from build123d import *

# Parameters (mm, degrees)
F0_R     = 63.5
F1_DEPTH = 63.5
F2_R     = 2.776459
F2_R_2   = 2.032
F2_R_3   = 3.5052
F3_DEPTH = 101.6


with BuildPart() as f1:
    # F0 (on Top) → F1 (new body, symmetric)
    with BuildSketch(Plane.XY):
        Circle(F0_R)
    extrude(amount=F1_DEPTH, both=True)

    # F2 (on face) → F3 (cut)
    with BuildSketch(Plane.XY.offset(63.5)):
        with BuildLine():
            ThreePointArc((-3.5052, 0), (0, -3.5052), (3.5052, 0))
            ThreePointArc((3.5052, 0), (0, 3.5052), (-3.5052, 0))
        make_face()
        with Locations((-47.625, 0)):
            Circle(F2_R)
        with BuildLine():
            ThreePointArc((-33.782, 0), (-31.75, -2.032), (-29.718, 0))
            Line((-29.718, 0), (-31.75, 0))
            Line((-31.75, 0), (-33.782, 0))
        make_face()
        with BuildLine():
            Line((-31.75, 0), (-29.718, 0))
            ThreePointArc((-29.718, 0), (-31.75, 2.032), (-33.782, 0))
            Line((-33.782, 0), (-31.75, 0))
        make_face()
        with BuildLine():
            ThreePointArc((-19.3802, 0), (-15.875, -3.5052), (-12.3698, 0))
            Line((-12.3698, 0), (-15.875, 0))
            Line((-15.875, 0), (-19.3802, 0))
        make_face()
        with BuildLine():
            Line((-15.875, 0), (-12.3698, 0))
            ThreePointArc((-12.3698, 0), (-15.875, 3.5052), (-19.3802, 0))
            Line((-19.3802, 0), (-15.875, 0))
        make_face()
        with Locations((-46.002217, -12.326257)):
            Circle(F2_R)
        with Locations((-41.24446, -23.8125)):
            Circle(F2_R)
        with Locations((-33.67596, -33.67596)):
            Circle(F2_R)
        with Locations((-23.8125, -41.24446)):
            Circle(F2_R)
        with Locations((-12.326257, -46.002217)):
            Circle(F2_R)
        with Locations((0, -47.625)):
            Circle(F2_R)
        with Locations((12.326257, -46.002217)):
            Circle(F2_R)
        with Locations((23.8125, -41.24446)):
            Circle(F2_R)
        with Locations((33.67596, -33.67596)):
            Circle(F2_R)
        with Locations((41.24446, -23.8125)):
            Circle(F2_R)
        with Locations((46.002217, -12.326257)):
            Circle(F2_R)
        with Locations((47.625, 0)):
            Circle(F2_R)
        with Locations((46.002217, 12.326257)):
            Circle(F2_R)
        with Locations((41.24446, 23.8125)):
            Circle(F2_R)
        with Locations((33.67596, 33.67596)):
            Circle(F2_R)
        with Locations((23.8125, 41.24446)):
            Circle(F2_R)
        with Locations((12.326257, 46.002217)):
            Circle(F2_R)
        with Locations((0, 47.625)):
            Circle(F2_R)
        with Locations((-12.326257, 46.002217)):
            Circle(F2_R)
        with Locations((-23.8125, 41.24446)):
            Circle(F2_R)
        with Locations((-33.67596, 33.67596)):
            Circle(F2_R)
        with Locations((-41.24446, 23.8125)):
            Circle(F2_R)
        with Locations((-46.002217, 12.326257)):
            Circle(F2_R)
        with Locations((-29.835241, -10.85914)):
            Circle(F2_R_2)
        with Locations((-24.321911, -20.408507)):
            Circle(F2_R_2)
        with Locations((-15.875, -27.496307)):
            Circle(F2_R_2)
        with Locations((-5.51333, -31.267646)):
            Circle(F2_R_2)
        with Locations((5.51333, -31.267646)):
            Circle(F2_R_2)
        with Locations((15.875, -27.496307)):
            Circle(F2_R_2)
        with Locations((24.321911, -20.408507)):
            Circle(F2_R_2)
        with Locations((29.835241, -10.85914)):
            Circle(F2_R_2)
        with Locations((31.75, 0)):
            Circle(F2_R_2)
        with Locations((29.835241, 10.85914)):
            Circle(F2_R_2)
        with Locations((24.321911, 20.408507)):
            Circle(F2_R_2)
        with Locations((15.875, 27.496307)):
            Circle(F2_R_2)
        with Locations((5.51333, 31.267646)):
            Circle(F2_R_2)
        with Locations((-5.51333, 31.267646)):
            Circle(F2_R_2)
        with Locations((-15.875, 27.496307)):
            Circle(F2_R_2)
        with Locations((-24.321911, 20.408507)):
            Circle(F2_R_2)
        with Locations((-29.835241, 10.85914)):
            Circle(F2_R_2)
        with Locations((-11.22532, -11.22532)):
            Circle(F2_R_3)
        with Locations((0, -15.875)):
            Circle(F2_R_3)
        with Locations((11.22532, -11.22532)):
            Circle(F2_R_3)
        with Locations((15.875, 0)):
            Circle(F2_R_3)
        with Locations((11.22532, 11.22532)):
            Circle(F2_R_3)
        with Locations((0, 15.875)):
            Circle(F2_R_3)
        with Locations((-11.22532, 11.22532)):
            Circle(F2_R_3)
    extrude(amount=-F3_DEPTH, mode=Mode.SUBTRACT)


solid = f1.part
Check sheet for the modelled part. Datum: model origin and axes. Units: mm. Round coordinates to 2 decimals unless told otherwise and drop trailing zeros. Order: outer loops, then holes, each group sorted by start corner. A loop starts at its lowest first (then second) coordinate and runs counter-clockwise, first axis right, second up. Notation, with made-up numbers: M 16,16.25 L 66,16.25 A21 cw 66,35.25 Z; hole C -22,69.25 d9. An arc over 180 degrees is marked long. One line per item, written item: value. Start each with the question number.
1. Gauge pin test, flat ends, axial feed: P1, Ø6, axis at x = -23, y = 42.5, coming from the +Z side; P2, Ø4.5, axis at x = 0, y = -47.625, coming from the +Z side; P3, Ø3, axis at x = -50.5, z = -47, coming from the +Y side; P4, Ø5, axis at y = -27, z = -29.5, coming from the -X side. Record the tip position at first contact, or that the pin passes through.
2. Section check A-A on x = 0. Enter the section's corners in (y, z).
3. Section check C-C on z = -44. Enter the section's corners in (x, y).
4. Section check D-D on z = 52. Give the number of separate pieces and of enclosed holes in the cut face, and give its area (3 significant figures).
5. Scan lines: line 1 along Y through (x, z) = (0, 12); line 2 along X through (y, z) = (-33.5, 24.5); line 3 along Y through (x, z) = (-15.5, 8.5). Record each from-to range of solid material in increasing order.
Results found:
1. P1: z = 63.5
1. P2: z = -38.1
1. P3: y = 40.39
1. P4: x = -58.58
2. outline: M -63.5,-63.5 L 63.5,-63.5 L 63.5,63.5 L 50.4,63.5 L 50.4,-38.1 L 44.85,-38.1 L 44.85,63.5 L 19.38,63.5 L 19.38,-38.1 L 12.37,-38.1 L 12.37,63.5 L 3.51,63.5 L 3.51,-38.1 L -3.51,-38.1 L -3.51,63.5 L -12.37,63.5 L -12.37,-38.1 L -19.38,-38.1 L -19.38,63.5 L -44.85,63.5 L -44.85,-38.1 L -50.4,-38.1 L -50.4,63.5 L -63.5,63.5 Z
3. outline: C 0,0 d127
4. separate pieces: 1
4. enclosed holes: 51
4. area: 11,500 mm^2
5. line 1: -63.5 to -50.4, -44.85 to -19.38, -12.37 to -3.51, 3.51 to 12.37, 19.38 to 44.85, 50.4 to 63.5
5. line 2: -53.94 to -36.45, -30.91 to 30.91, 36.45 to 53.94
5. line 3: -61.58 to -29.49, -25.5 to -3.49, 3.49 to 25.5, 29.49 to 61.58
